The figure shows three views and two pictorial views of one solid part (mm, origin at its lowest corner). Answer the questions. Give positions to 0.01 mm unless a question says otherwise; leave off trailing zeros. Write each loop counter-clockwise with the first axis right and the second up, starting at its lowest first coordinate (ties: lowest second). Pieces come first, ordered by that corner, then holes. Notation, with made-up numbers: (11, -34.75) - (52, -34.75) arc R24 cw to (52, -23.75) - close; hole circle Ø2 at (77, -26). An arc over 180 degrees is marked (long way). Answer as CSV lines item,"result". Start each with the question number.
(1) Find section C-C (x = 273). Write down the section's boundary in (y, z).
(2) Find section D-D (x = 52.5). Write down the section's boundary in (y, z).
(3) Each of these flat-tipped pins is pushed along its axis until it touches: pin 1 Ø6 at (x, y) = (86.5, 15.5) entering from +Z; pin 2 Ø5 at (x, z) = (98.5, 41.5) entering from -Y; pin 3 Ø6 at (x, z) = (45, 8.5) entering from -Y. Where does it stop, or does it pass through?
(4) Find section B-B (z = 16). Write down the section's boundary in (x, y), then the cut area to 3 significant figures.
(5) Straight lines are drawn through the part: probe 1 along X at (y, z) = (27, 35); probe 2 along X at (y, z) = (28.5, 28); probe 3 along Y at (x, z) = (342, 24). For each, find the intervals that lie inside material, in ascending order.
(6) Find section A-A (z = 51). Write down the section's boundary in (x, y), then the cut area to 3 significant figures.
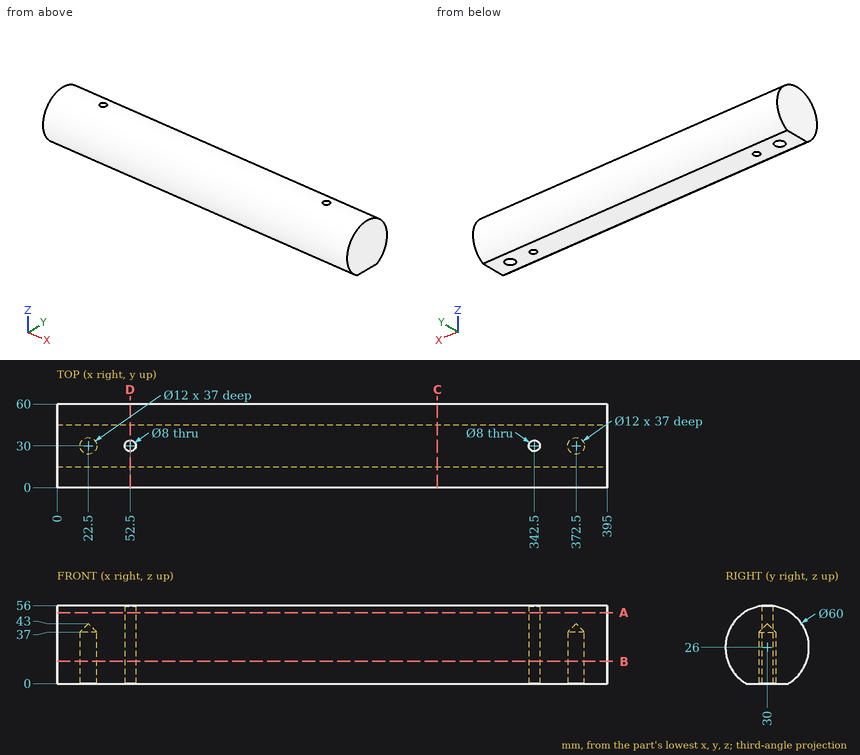
Result set:
1,outline,"(15.03, 0) - (44.97, 0) arc R30 ccw (long way) to start"
2,outline,"(15.03, 0) - (26, 0) - (26, 55.73) arc R30 ccw to start; (34, 0) - (44.97, 0) arc R30 ccw to (34, 55.73) - close"
3,pin 1,"z = 53.71"
3,pin 2,"y = 2.96"
3,pin 3,"y = 3.74"
4,outline,"(0, 1.72) - (395, 1.72) - (395, 58.28) - (0, 58.28) - close; hole circle Ø12 at (22.5, 30); hole circle Ø8 at (52.5, 30); hole circle Ø8 at (342.5, 30); hole circle Ø12 at (372.5, 30)"
4,area,"22,000 mm^2"
5,probe 1,"0 to 17.3, 27.7 to 49.85, 55.15 to 339.85, 345.15 to 367.3, 377.7 to 395"
5,probe 2,"0 to 16.69, 28.31 to 48.79, 56.21 to 338.79, 346.21 to 366.69, 378.31 to 395"
5,probe 3,"0.07 to 26.03, 33.97 to 59.93"
6,outline,"(0, 13.42) - (395, 13.42) - (395, 46.58) - (0, 46.58) - close; hole circle Ø8 at (52.5, 30); hole circle Ø8 at (342.5, 30)"
6,area,"13,000 mm^2"
